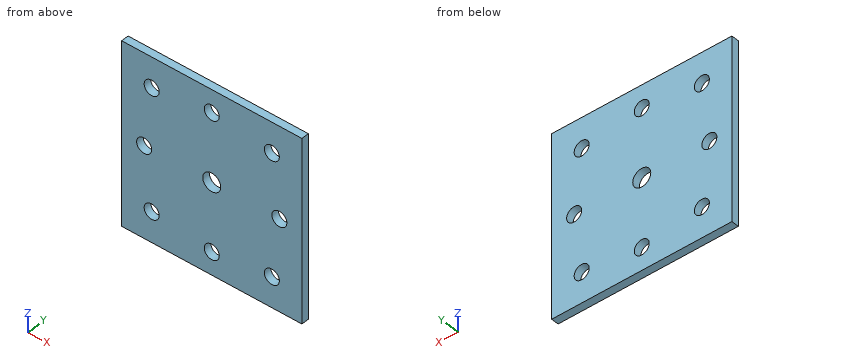
Autodesk Inventor part; units mm, degrees
ref_plane "YZ Plane" through (0, 0, 0) normal (1, 0, 0) x (0, 1, 0)
ref_plane "XZ Plane" through (0, 0, 0) normal (0, 1, 0) x (-1, 0, 0)
ref_plane "XY Plane" through (0, 0, 0) normal (0, 0, 1) x (1, 0, 0)
sketch "Sketch1" plane through (0, 0, 0) normal (0, 1, 0) x (-1, 0, 0)
  line L0 (0, 0) -> (-76.2, 0)
  line L1 (-76.2, 0) -> (-76.2, -76.2)
  line L2 (-76.2, -76.2) -> (0, -76.2)
  line L3 (0, -76.2) -> (0, 0)
  dimension "d0" = 76.2
  dimension "d1" = 76.2
extrude "Extrusion1" add sketch "Sketch1" along normal blind 3.175
sketch "Sketch2" plane through (0, 3.175, 0) normal (0, 1, 0) x (1, 0, 0)
  line L0 (76.2, 76.2) -> (0, 76.2)
  line L1 (0, 76.2) -> (0, 0)
  line L2 (9.525, 38.1) -> (38.1, 66.675)
  line L3 (38.1, 66.675) -> (66.675, 38.1)
  line L4 (66.675, 38.1) -> (38.1, 9.525)
  line L5 (38.1, 9.525) -> (9.525, 38.1)
  line L6 (0, 0) -> (76.2, 0)
  dimension "d5" = 57.15
  dimension "d7" = 57.15
  dimension "d8" = 9.525
  dimension "d9" = 9.525
  dimension "d29" = 45
hole "Hole1" at (38.1, 3.175, -66.675) at (9.525, 3.175, -38.1) at (38.1, 3.175, -9.525) at (66.675, 3.175, -38.1) direction (0, -1, 0) diameter 6.35 end through all
sketch "Sketch3" plane through (0, 3.175, 0) normal (0, 1, 0) x (1, 0, 0)
  line L0 (76.2, 0) -> (76.2, 76.2)
  line L1 (76.2, 76.2) -> (0, 76.2)
  line L2 (12.7, 63.5) -> (63.5, 63.5)
  line L3 (63.5, 63.5) -> (63.5, 12.7)
  line L4 (63.5, 12.7) -> (12.7, 12.7)
  line L5 (12.7, 12.7) -> (12.7, 63.5)
  dimension "d17" = 50.8
  dimension "d19" = 50.8
  dimension "d20" = 12.7
  dimension "d21" = 12.7
hole "Hole2" at (12.7, 3.175, -63.5) at (63.5, 3.175, -63.5) at (12.7, 3.175, -12.7) at (63.5, 3.175, -12.7) direction (0, -1, 0) diameter 6.35 end through all
sketch "Sketch4" plane through (0, 3.175, 0) normal (0, 1, 0) x (1, 0, 0)
  line L0 (0, 0) -> (76.2, 0)
  line L1 (76.2, 0) -> (76.2, 76.2)
  point P0 (38.1, 38.1)
  dimension "d34" = 38.1
  dimension "d35" = 38.1
hole "Hole3" at (38.1, 3.175, -38.1) direction (0, -1, 0) diameter 7.62 end through all
properties part number "CouplerBridge"
Can you work these out from the model? Positions are in its coordinate system, mm. Give positions to 0.01 mm unless a question says otherwise; leave off trailing zeros. Order: outer loops, then holes, each group sorted by start corner. A loop starts at its lowest first (then second) coordinate and runs counter-clockwise, first axis right, second up. Notation, with made-up numbers: (0.25, -34) - (22.25, -34) arc R30 cw to (22.25, -9) - close; hole circle Ø9 at (47.5, 49.5). An arc over 180 degrees is marked (long way). Use a Markdown table: item, result. Add a question column.
Q1. Please list where these lines run through material, in increasing order: line 1 along X through (y, z) = (2.1, -13); line 2 along Z through (x, y) = (38.1, 0.7); line 3 along Z through (x, y) = (10, 0.8).
Q2. If we section it at A-A on z = -38.1: Write out the boundary of the cut face in (x, y) (3 decimals), plus the area to 3 significant figures.
Q3. If we section it at C-C on x = 38.1: Write out the boundary of the cut face in (y, z) (3 decimals), plus the area to 3 significant figures.
Q4. If we section it at B-B on y = 1.2: Count the separate pieces of the cut face and the enclosed holes in it, plus the area to 3 significant figures.
Answers follow:
| question | item | result |
|---|---|---|
| 1 | line 1 | x = 0 to 9.54, 15.86 to 60.34, 66.66 to 76.2 |
| 1 | line 2 | z = -76.2 to -69.85, -63.5 to -41.91, -34.29 to -12.7, -6.35 to 0 |
| 1 | line 3 | z = -76.2 to -65.17, -61.83 to -41.24, -34.96 to -14.37, -11.03 to 0 |
| 2 | outline | (0, 0) - (6.35, 0) - (6.35, 3.175) - (0, 3.175) - close; (12.7, 0) - (34.29, 0) - (34.29, 3.175) - (12.7, 3.175) - close; (41.91, 0) - (63.5, 0) - (63.5, 3.175) - (41.91, 3.175) - close; (69.85, 0) - (76.2, 0) - (76.2, 3.175) - (69.85, 3.175) - close |
| 2 | area | 177 mm^2 |
| 3 | outline | (0, -76.2) - (3.175, -76.2) - (3.175, -69.85) - (0, -69.85) - close; (0, -63.5) - (3.175, -63.5) - (3.175, -41.91) - (0, -41.91) - close; (0, -34.29) - (3.175, -34.29) - (3.175, -12.7) - (0, -12.7) - close; (0, -6.35) - (3.175, -6.35) - (3.175, 0) - (0, 0) - close |
| 3 | area | 177 mm^2 |
| 4 | separate pieces | 1 |
| 4 | enclosed holes | 9 |
| 4 | area | 5,510 mm^2 |
